```python
from build123d import *

# Parameters (mm, degrees)
BOSS_EXTRUDE1_DEPTH = 41.402
SKETCH2_R           = 2.0193
CUT_EXTRUDE2_DEPTH  = 12.7
SKETCH3_R           = 1.842835094
CUT_EXTRUDE7_DEPTH  = 12.7


with BuildPart() as part:
    # Sketch1 → Boss-Extrude1 (new body)
    with BuildSketch(Plane.XY):
        Polygon((3.242368481, 6.576502107), (-4.074233653, 6.096224526), (-7.316602133, -0.480277581), (-3.242368481, -6.576502107), (4.074233653, -6.096224526), (7.316602133, 0.480277581), align=None)
    extrude(amount=BOSS_EXTRUDE1_DEPTH)

    # Sketch2 → Cut-Extrude2 (cut)
    with BuildSketch(Plane.XY.offset(41.402)):
        with Locations((0.049397867, 0.013636683)):
            Circle(SKETCH2_R)
    extrude(amount=-CUT_EXTRUDE2_DEPTH, mode=Mode.SUBTRACT)

    # Sketch3 → Cut-Extrude7 (cut)
    with BuildSketch(Plane(origin=(0, 0, 0), x_dir=(-1, 0, 0), z_dir=(0, 0, -1))):
        with Locations((0.049397867, -0.003242583)):
            Circle(SKETCH3_R)
    extrude(amount=-CUT_EXTRUDE7_DEPTH, mode=Mode.SUBTRACT)


solid = part.part
```
Model file for the job. Use its own axes, mm. A direction names the side the tool comes from. Coordinates: 2 decimals unless noted, no trailing zeros. Loops run counter-clockwise (first coordinate to the right, second up) from the corner with the lowest first, then second, coordinate; pieces in that order, holes last. Notation, with made-up numbers: M -22.5,-31 L 2.5,-31 A19 cw 2.5,-5 Z; hole C 5,52 d5. An arc over 180 degrees is marked long. Use CSV: the item, a comma, the result in double quotes. Start each with the question number.
1. Band-saw the part on A-A, the plane z = 5. List the corners of the cut face in (x, y), then the cut area to 3 significant figures.
2. Tool access for faces 1 (the cylindrical face through (1.975, 0.62, 35.141)), 2 (the cylindrical face through (-1.807, 0.55, 6.261)), 3 (the flat face through (2, -1, 41.402)): list every direction of +Z, -Z, +X, -X, +Y, -Y with a clear straight run to the whole face (end or side of a thin tool).
3. Probe probe 1 along Z at (x, y) = (-1, -1.5); probe 2 along X at (y, z) = (-1.5, 11); probe 3 along Y at (x, z) = (-3.25, 17). List the from-to ranges inside material, lowest first. Write a range as [from, to].
4. Flat gauge pins, fed straight in: pin 1 (4 mm diameter, centred on y = -4.5, z = 8.5, fed in from +X); pin 2 (2.5 mm diameter, centred on x = 0.05, y = 0.01, fed in from +Z); pin 3 (1.1 mm diameter, centred on x = -1, y = 1, fed in from -Z); pin 4 (1.5 mm diameter, centred on x = 1, z = 31.5, fed in from -Y). Where does each tip first touch, or does it go through?
5. Band-saw the part on B-B, the plane x = 0.5. List the corners of the cut face in (y, z), then the cut area to 3 significant figures.
6. Band-saw the part on C-C, the plane y = -1. List the corners of the cut face in (x, z), then the cut area to 3 significant figures.
7. Two-plate mould, pull along X, no slides. Class faces 4 (the flat face through (5.3, 3.5, 20.4)), 5 (the flat face through (-5.3, -3.5, 20.4)), 6 (the flat face through (0, 0, 28.702)), 7 (the flat face through (0, 0, 12.7)): pulls with the +X half, pulls with the -X half, needs draft (parallel to the pull), parting line crosses it, or undercut.
8. Band-saw the part on D-D, the plane z = 22. List the corners of the cut face in (x, y), then the cut area to 3 significant figures.
Entries:
1,outline,"M -7.32,-0.48 L -3.24,-6.58 L 4.07,-6.1 L 7.32,0.48 L 3.24,6.58 L -4.07,6.1 Z; hole C -0.05,0 d3.69"
1,area,"129 mm2"
2,face 1,"+Z"
2,face 2,"-Z"
2,face 3,"+Z, +X, -X, +Y, -Y"
3,probe 1,"z = [12.7, 28.7]"
3,probe 2,"x = [-6.64, -1.12], [1.03, 6.34]"
3,probe 3,"y = [-6.57, 6.15]"
4,pin 1,"stops at x = 5.85"
4,pin 2,"stops at z = 28.7"
4,pin 3,"stops at z = 0"
4,pin 4,"stops at y = -6.35"
5,outline,"M -6.33,0 L -1.76,0 L -1.76,12.7 L 1.76,12.7 L 1.76,0 L 6.4,0 L 6.4,41.4 L 1.98,41.4 L 1.98,28.7 L -1.95,28.7 L -1.95,41.4 L -6.33,41.4 Z"
5,area,"432 mm2"
6,outline,"M -6.97,0 L -1.6,0 L -1.6,12.7 L 1.5,12.7 L 1.5,0 L 6.59,0 L 6.59,41.4 L 1.8,41.4 L 1.8,28.7 L -1.7,28.7 L -1.7,41.4 L -6.97,41.4 Z"
6,area,"478 mm2"
7,face 4,"pulls with the +X half"
7,face 5,"pulls with the -X half"
7,face 6,"undercut"
7,face 7,"undercut"
8,outline,"M -7.32,-0.48 L -3.24,-6.58 L 4.07,-6.1 L 7.32,0.48 L 3.24,6.58 L -4.07,6.1 Z"
8,area,"140 mm2"
